from build123d import *

# Parameters (mm, degrees)
EXTRUDE1_DEPTH = 16
EXTRUDE6_DEPTH = 12
SKETCH3_R      = 1.5
EXTRUDE7_DEPTH = 4
FILLET1_R      = 3
FILLET2_R      = 3


with BuildPart() as part:
    # Sketch1 → Extrude1 (new body)
    with BuildSketch(Plane.XY):
        Polygon((16.5, -10.5), (25, -10.5), (25, -14.5), (-25, -14.5), (-25, -10.5), (-16.5, -10.5), (-16.5, 14.5), (16.5, 14.5), align=None)
    extrude(amount=-EXTRUDE1_DEPTH)

    # Sketch2 → Extrude6 (cut)
    with BuildSketch(Plane.XY):
        Polygon((1, 14.5), (-1, 14.5), (-1, 4.5), (-16.5, 4.5), (-16.5, 2.5), (16.5, 2.5), (16.5, 4.5), (1, 4.5), align=None)
    extrude(amount=-EXTRUDE6_DEPTH, mode=Mode.SUBTRACT)

    # Sketch3 → Extrude7 (cut)
    with BuildSketch(Plane.XZ.offset(14.5)):
        with Locations((-20.5, -8)):
            Circle(SKETCH3_R)
        with Locations((20.5, -8)):
            Circle(SKETCH3_R)
    extrude(amount=-EXTRUDE7_DEPTH, mode=Mode.SUBTRACT)

    # Fillet1
    fillet1_edges = [part.edges().sort_by_distance(p)[0] for p in [
        (-1, 9.5, 0),
        (8.75, 4.5, 0),
        (-8.75, 4.5, 0),
        (0, 2.5, 0),
        (1, 9.5, 0),
    ]]
    fillet(fillet1_edges, radius=FILLET1_R)

    # Fillet2
    fillet2_edges = [part.edges().sort_by_distance(p)[0] for p in [
        (-25, -12.5, 0),
        (-16.5, 2, -16),
        (-25, -12.5, -16),
        (25, -12.5, -16),
        (16.5, 2, -16),
        (25, -12.5, 0),
    ]]
    fillet(fillet2_edges, radius=FILLET2_R)


solid = part.part
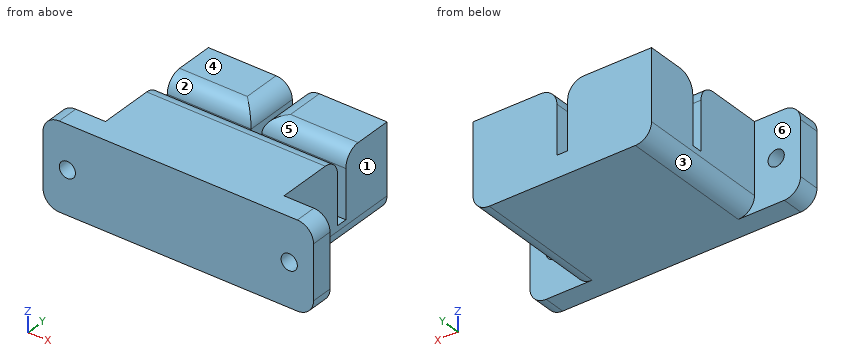
Read the model definition and answer for the solid it produces. Units are mm, in the model's axes. Face numbers are marked on the shaded views. A direction names the side the tool comes from. Give positions to 0.01 mm unless a question says otherwise; leave off trailing zeros. Loops run counter-clockwise (first coordinate to the right, second up) from the corner with the lowest first, then second, coordinate; pieces in that order, holes last. Notation, with made-up numbers: (55, 44) - (100, 44) arc R19 ccw to (100, 49) - close; hole circle Ø3 at (26.5, 0). An arc over 180 degrees is marked (long way). Answer as CSV lines item,"result". Start each with the question number.
1) Each of these flat-tipped pins is pushed along its axis until it touches: pin 1 Ø3 at (y, z) = (-7, -11.5) entering from -X; pin 2 Ø5 at (y, z) = (6.5, -10.5) entering from +X; pin 3 Ø6 at (x, z) = (21.5, -5.5) entering from +Y. Where does it stop, or does it pass through?
2) Determine the mould class of the marked faces 4, 5 and 6 for opening direction Y: released by +Y, released by -Y, zero draft, split by the parting line, or undercut.
3) Find section C-C (z = -4). Write down the section's boundary in (x, y).
4) Find section B-B (z = -8). Write down the section's boundary in (x, y).
5) Which of the six approach directions +Z, -Z, +X, -X, +Y, -Y give full straight-line access (tool end or side, diameter ignored) to the marked faces 1, 2 and 3?
6) Find section D-D (y = -7.5). Write down the section's boundary in (x, z).
7) Straight lines are drawn through the part: L1, parallel to X at y = 11.25, z = -4.75; L2, parallel to Y at x = -7, z = -2.75; L3, parallel to Z at x = 20.5, y = -11.85. For each, find the intervals that lie inside material, in ascending order. Write a range as from..to.
8) Find section A-A (x = 20.5). Write down the section's boundary in (y, z).
Findings below:
1,pin 1,"x = -16.5"
1,pin 2,"x = 16.5"
1,pin 3,"y = -10.5"
2,face 4,"zero draft"
2,face 5,"undercut"
2,face 6,"released by +Y"
3,outline,"(-25, -14.5) - (25, -14.5) - (25, -10.5) - (16.5, -10.5) - (16.5, 2.5) - (-16.5, 2.5) - (-16.5, -10.5) - (-25, -10.5) - close; (-16.5, 4.5) - (-1, 4.5) - (-1, 14.5) - (-16.5, 14.5) - close; (1, 4.5) - (16.5, 4.5) - (16.5, 14.5) - (1, 14.5) - close"
4,outline,"(-25, -14.5) - (-22, -14.5) - (-22, -10.5) - (-25, -10.5) - close; (-19, -14.5) - (19, -14.5) - (19, -10.5) - (16.5, -10.5) - (16.5, 2.5) - (-16.5, 2.5) - (-16.5, -10.5) - (-19, -10.5) - close; (-16.5, 4.5) - (-1, 4.5) - (-1, 14.5) - (-16.5, 14.5) - close; (1, 4.5) - (16.5, 4.5) - (16.5, 14.5) - (1, 14.5) - close; (22, -14.5) - (25, -14.5) - (25, -10.5) - (22, -10.5) - close"
5,face 1,"+Z, -Z, +X, +Y"
5,face 2,"+Z, +X, -X"
5,face 3,"-Z, -X, +Y"
6,outline,"(-16.5, -13) arc R3 ccw to (-13.5, -16) - (13.5, -16) arc R3 ccw to (16.5, -13) - (16.5, 0) - (-16.5, 0) - close"
7,L1,"-16.5..-1, 1..16.5"
7,L2,"-14.5..2.49, 4.51..14.5"
7,L3,"-16..-9.5, -6.5..0"
8,outline,"(-14.5, -16) - (-10.5, -16) - (-10.5, -9.5) - (-14.5, -9.5) - close; (-14.5, -6.5) - (-10.5, -6.5) - (-10.5, 0) - (-14.5, 0) - close"
